The model under review builds one solid part; all positions refer to its coordinate system, in mm. A direction names the side the tool comes from. Round coordinates to 2 decimals unless told otherwise and drop trailing zeros. Loops run counter-clockwise (first coordinate to the right, second up) from the corner with the lowest first, then second, coordinate; pieces in that order, holes last. Notation, with made-up numbers: M 62.5,38 L 98.5,38 A15 cw 98.5,61 Z; hole C 89.25,19 d1. An arc over 180 degrees is marked long. Answer in a Markdown table with one row per item. Add a question column.
from build123d import *

# Parameters (mm, degrees)
SKETCH1_W                       = 76.2
SKETCH1_H                       = 19.05
BOSS_EXTRUDE1_DEPTH             = 9.525
FILLET1_R                       = 2
BOSS_EXTRUDE2_DEPTH             = 2
BOSS_EXTRUDE2_DIRECTION_2_REACH = 79.381


with BuildPart() as part:
    # Sketch1 → Boss-Extrude1 (new, symmetric)
    with BuildSketch(Plane(origin=(0, 0, 0), x_dir=(0, 0, -1), z_dir=(1, 0, 0))):
        Rectangle(SKETCH1_W, SKETCH1_H)
    extrude(amount=BOSS_EXTRUDE1_DEPTH, both=True)

    # Fillet1
    fillet1_edges = [part.edges().sort_by_distance(p)[0] for p in [
        (9.525, 0, 38.1),
        (9.525, -9.525, 0),
        (9.525, 0, -38.1),
        (-9.525, -9.525, 0),
        (-9.525, 0, 38.1),
        (-9.525, 9.525, 0),
        (-9.525, 0, -38.1),
        (0, -9.525, -38.1),
        (0, -9.525, 38.1),
        (0, 9.525, 38.1),
        (0, 9.525, -38.1),
        (9.525, 9.525, 0),
    ]]
    fillet(fillet1_edges, radius=FILLET1_R)

    # Sketch2 → Boss-Extrude2 (add)
    with BuildSketch(Plane(origin=(0, 0, -38.1), x_dir=(-1, 0, 0), z_dir=(0, 0, -1))):
        with BuildLine():
            Line((-5.771898524, 9.525), (5.739747172, 9.525))
            ThreePointArc((5.739747172, 9.525), (8.406747172, 6.858), (5.739747172, 4.191))
            Line((5.739747172, 4.191), (-5.771898524, 4.191))
            ThreePointArc((-5.771898524, 4.191), (-8.438898524, 6.858), (-5.771898524, 9.525))
        make_face()
    extrude(amount=BOSS_EXTRUDE2_DEPTH)

    # Sketch2 → Boss-Extrude2 direction 2 (add, up to next)
    with BuildSketch(Plane(origin=(0, 0, -38.1), x_dir=(-1, 0, 0), z_dir=(0, 0, -1)), mode=Mode.PRIVATE) as boss_extrude2_direction_2_sk1:
        with BuildLine():
            Line((-5.771898524, 9.525), (5.739747172, 9.525))
            ThreePointArc((5.739747172, 9.525), (8.406747172, 6.858), (5.739747172, 4.191))
            Line((5.739747172, 4.191), (-5.771898524, 4.191))
            ThreePointArc((-5.771898524, 4.191), (-8.438898524, 6.858), (-5.771898524, 9.525))
        make_face()
    boss_extrude2_direction_2_tool1 = extrude(boss_extrude2_direction_2_sk1.sketch, amount=-BOSS_EXTRUDE2_DIRECTION_2_REACH, mode=Mode.PRIVATE) - part.part
    add(boss_extrude2_direction_2_tool1.solids().sort_by_distance((0.016076, 6.858, -38.1))[0])


solid = part.part
1. Take a section at A-A, the plane y = 0. State the section outline as (x, z) points (3 decimals).
2. Machinability: for faces 1 (the cylindrical face through (7.03, 9.47, -36.57)), 2 (the cylindrical face through (-8.406, 6.917, -39.017)), 3 (the cylindrical face through (-8.924, 0.105, -37.53)), 4 (the cylindrical face through (8.44, 6.8, -39.02)), which of the approach directions +Z, -Z, +X, -X, +Y, -Y give a long, thin tool a straight path to every point of the face, cutting with its end or side? Answer none if there is none.
3. Take a section at C-C, the plane x = -6.75. State the section outline as (y, z) points (3 decimals), and give its area (3 significant figures).
4. Take a section at B-B, the plane x = 1. State the section outline as (y, z) points (3 decimals).
5. For pin 1 Ø1 at (x, z) = (2.5, -39) entering from -Y, flat-tipped, find the tip position at first contact; note if it passes through.
6. To check wall thickness, follow probe 1 along Z at (x, y) = (0.25, -6); probe 2 along X at (y, z) = (8.25, 11.5); probe 3 along Z at (x, y) = (4.75, 8.5). State the ranges of each line that lie inside material, in increasing order.
Check sheet entries:
| question | item | result |
|---|---|---|
| 1 | outline | M -9.525,-36.1 A2 ccw -7.525,-38.1 L 7.525,-38.1 A2 ccw 9.525,-36.1 L 9.525,36.1 A2 ccw 7.525,38.1 L -7.525,38.1 A2 ccw -9.525,36.1 Z |
| 2 | face 1 | -Z, +X, +Y |
| 2 | face 2 | -Z, -X |
| 2 | face 3 | -Z, -X, -Y |
| 2 | face 4 | -Z, +X |
| 3 | outline | M -9.525,-36.1 A2 ccw -7.525,-38.1 L 4.39,-38.1 L 4.39,-40.1 L 9.326,-40.1 L 9.326,-36.969 A2 ccw 9.525,-36.1 L 9.525,36.1 A2 ccw 7.525,38.1 L -7.525,38.1 A2 ccw -9.525,36.1 Z |
| 3 | area | 1,460 mm^2 |
| 4 | outline | M -9.525,-36.1 A2 ccw -7.525,-38.1 L 4.191,-38.1 L 4.191,-40.1 L 9.525,-40.1 L 9.525,36.1 A2 ccw 7.525,38.1 L -7.525,38.1 A2 ccw -9.525,36.1 Z |
| 5 | pin 1 | stops at y = 4.19 |
| 6 | probe 1 | z = -38.1 to 38.1 |
| 6 | probe 2 | x = -9.39 to 9.39 |
| 6 | probe 3 | z = -40.1 to 37.85 |
